```python
from build123d import *

# Parameters (mm, degrees)
BOSS_EXTRUDE1_DEPTH      = 25.4
BOSS_EXTRUDE1_DEPTH_BACK = 34.925
CUT_EXTRUDE4_DEPTH       = 61.325
CUT_EXTRUDE5_DEPTH       = 26.4
SKETCH14_R               = 3.2893
CUT_EXTRUDE6_DEPTH       = 26.4


with BuildPart() as part:
    # Sketch1 → Boss-Extrude1 (new body, two sides)
    with BuildSketch(Plane(origin=(0, 0, 0), x_dir=(0, 0, -1), z_dir=(1, 0, 0))) as boss_extrude1_sk:
        with BuildLine():
            Line((-10.16, 12.7), (10.16, 12.7))
            ThreePointArc((10.16, 12.7), (11.956051224, 11.956051224), (12.7, 10.16))
            Line((12.7, 10.16), (12.7, -10.16))
            ThreePointArc((12.7, -10.16), (11.956051224, -11.956051224), (10.16, -12.7))
            Line((10.16, -12.7), (-10.16, -12.7))
            ThreePointArc((-10.16, -12.7), (-11.956051224, -11.956051224), (-12.7, -10.16))
            Line((-12.7, -10.16), (-12.7, 10.16))
            ThreePointArc((-12.7, 10.16), (-11.956051224, 11.956051224), (-10.16, 12.7))
        make_face()
    extrude(amount=BOSS_EXTRUDE1_DEPTH)
    extrude(boss_extrude1_sk.sketch, amount=-BOSS_EXTRUDE1_DEPTH_BACK)

    # Sketch11 → Cut-Extrude4 (cut, through all)
    with BuildSketch(Plane(origin=(25.4, 0, 0), x_dir=(0, 0, -1), z_dir=(1, 0, 0))):
        with BuildLine():
            Line((-10.6045, 11.1125), (10.6045, 11.1125))
            ThreePointArc((10.6045, 11.1125), (10.963710245, 10.963710245), (11.1125, 10.6045))
            Line((11.1125, 10.6045), (11.1125, -10.6045))
            ThreePointArc((11.1125, -10.6045), (10.963710245, -10.963710245), (10.6045, -11.1125))
            Line((10.6045, -11.1125), (-10.6045, -11.1125))
            ThreePointArc((-10.6045, -11.1125), (-10.963710245, -10.963710245), (-11.1125, -10.6045))
            Line((-11.1125, -10.6045), (-11.1125, 10.6045))
            ThreePointArc((-11.1125, 10.6045), (-10.963710245, 10.963710245), (-10.6045, 11.1125))
        make_face()
    extrude(amount=-CUT_EXTRUDE4_DEPTH, mode=Mode.SUBTRACT)

    # Sketch12 → Cut-Extrude5 (cut, through all)
    with BuildSketch(Plane(origin=(0, 12.7, 0), x_dir=(1, 0, 0), z_dir=(0, 1, 0))):
        with BuildLine():
            Line((0, 12.7), (50.8, 12.7))
            Line((50.8, 12.7), (50.8, -12.7))
            Line((50.8, -12.7), (0, -12.7))
            Line((0, -12.7), (19.444424463, -7.686083637))
            ThreePointArc((19.444424463, -7.686083637), (25.4, 0), (19.444424463, 7.686083637))
            Line((19.444424463, 7.686083637), (0, 12.7))
        make_face()
    extrude(amount=-CUT_EXTRUDE5_DEPTH, mode=Mode.SUBTRACT)

    # Sketch14 → Cut-Extrude6 (cut, through all)
    with BuildSketch(Plane(origin=(0, 12.7, 0), x_dir=(1, 0, 0), z_dir=(0, 1, 0))):
        with Locations((17.4625, 0)):
            Circle(SKETCH14_R)
    extrude(amount=-CUT_EXTRUDE6_DEPTH, mode=Mode.SUBTRACT)


solid = part.part
```
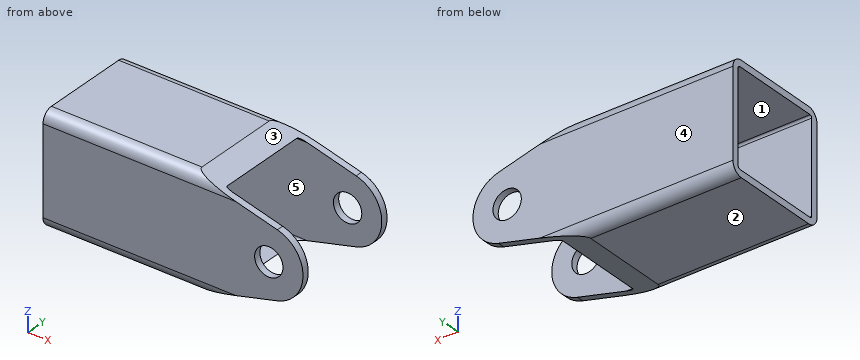
Design review of the part built by this model. Coordinates are the model's own, in mm. Face numbers are marked on the shaded views. A direction names the side the tool comes from. Round coordinates to 2 decimals unless told otherwise and drop trailing zeros. Write each loop counter-clockwise with the first axis right and the second up, starting at its lowest first coordinate (ties: lowest second). Pieces come first, ordered by that corner, then holes. Notation, with made-up numbers: (74.25, -39) -> (101.25, -39) arc R31 cw to (101.25, -13) -> close; hole circle Ø6 at (-27.75, -35). An arc over 180 degrees is marked (long way). Write item = value, one per line. Start each with the question number.
1) Mouldability with a two-part tool opening along Z and no side actions: class the marked faces 1, 2 and 3 as +Z half, -Z half, draft (parallel to the pull), parting line (faces both ways), or undercut.
2) Take a section at A-A, the plane y = 5.5. State the section outline as (x, z) points (1 decimal).
3) Take a section at C-C, the plane x = 2.5. State the section outline as (y, z) points, plus the area to 3 significant figures.
4) Take a section at D-D, the plane x = 10.5. State the section outline as (y, z) points.
5) Tool access review of the marked faces 4 and 5: name each direction out of +Z, -Z, +X, -X, +Y, -Y from which nothing blocks a thin tool from reaching the whole face with its end or side.
6) Clearance check with flat-ended pins moving along their axes: pin 1 (5 mm diameter, centred on y = -8.5, z = -2.5, fed in from -X); pin 2 (3 mm diameter, centred on x = 2, y = -7, fed in from -Z). State where each tip first meets the part, or that it passes through.
7) Wall thickness on probe 1 along Y at (x, z) = (-19, -0.25); probe 2 along Z at (x, y) = (2, 1.25): over which ranges is each line inside the solid? List them lowest first. Write a range as from..to.
8) Take a section at B-B, the plane z = 0. State the section outline as (x, y) points (1 decimal).
Results list:
q1.face_1 = undercut
q1.face_2 = -Z half
q1.face_3 = +Z half
q2.outline = (-34.9, -12.7) -> (0, -12.7) -> (6.2, -11.1) -> (-34.9, -11.1) -> close; (-34.9, 11.1) -> (6.2, 11.1) -> (0, 12.7) -> (-34.9, 12.7) -> close
q3.outline = (-12.7, -10.16) arc R2.54 ccw to (-11.85, -12.06) -> (11.85, -12.06) arc R2.54 ccw to (12.7, -10.16) -> (12.7, 10.16) arc R2.54 ccw to (11.85, 12.06) -> (-11.85, 12.06) arc R2.54 ccw to (-12.7, 10.16) -> close; hole (-11.11, -10.6) arc R0.51 ccw to (-10.6, -11.11) -> (10.6, -11.11) arc R0.51 ccw to (11.11, -10.6) -> (11.11, 10.6) arc R0.51 ccw to (10.6, 11.11) -> (-10.6, 11.11) arc R0.51 ccw to (-11.11, 10.6) -> close
q3.area = 117 mm²
q4.outline = (-12.7, -9.99) -> (-11.11, -9.99) -> (-11.11, 9.99) -> (-12.7, 9.99) -> close; (11.11, -9.99) -> (12.7, -9.99) -> (12.7, 9.99) -> (11.11, 9.99) -> close
q5.face_4 = +Z, -Z, +X, -X, +Y
q5.face_5 = +X, -X
q6.pin_1 = through
q6.pin_2 = -12.57
q7.probe_1 = -12.7..-11.11, 11.11..12.7
q7.probe_2 = -12.18..-11.11, 11.11..12.18
q8.outline = (-34.9, -12.7) -> (14.2, -12.7) -> (14.2, -11.1) -> (-34.9, -11.1) -> close; (-34.9, 11.1) -> (14.2, 11.1) -> (14.2, 12.7) -> (-34.9, 12.7) -> close; (20.8, -12.7) -> (25.4, -12.7) -> (25.4, -11.1) -> (20.8, -11.1) -> close; (20.8, 11.1) -> (25.4, 11.1) -> (25.4, 12.7) -> (20.8, 12.7) -> close
